```python
from build123d import *

# Parameters (mm, degrees)
F2_SIZE = 5
F3_R    = 0.99999


# Not quite as in the source:
# - a fillet or chamfer is up to 0.001 mm smaller than in the source, because OpenCascade refuses the exact size


with BuildPart() as f1:
    # F0 (on Front) → F1 (revolve)
    with BuildSketch(Plane.XZ):
        with BuildLine():
            Line((-2.5, -3), (-2.5, 0))
            Line((-2.5, 0), (-2.5, 15))
            Line((-2.5, 15), (-8, 15))
            ThreePointArc((-8, 15), (-11.5355339059, 13.5355339059), (-13, 10))
            Line((-13, 10), (-13, 8))
            Line((-13, 8), (-12, 8))
            ThreePointArc((-12, 8), (-8.4644660941, 6.5355339059), (-7, 3))
            ThreePointArc((-7, 3), (-7.8786796564, 0.8786796564), (-10, 0))
            Line((-10, 0), (-10.5, 0))
            Line((-10.5, 0), (-10.5, -3))
            Line((-10.5, -3), (-2.5, -3))
        make_face()
    revolve(axis=Axis((0, 0, 3.244361095), (0, 0, -1)))

    # F2
    f2_edges = [f1.edges().sort_by_distance(p)[0] for p in [
        (2.5, 0, 15),
    ]]
    chamfer(f2_edges, length=F2_SIZE)

    # F3 (radius 1 in the source; OpenCascade refuses exactly that, so slightly less here)
    f3_edges = [f1.edges().sort_by_distance(p)[0] for p in [
        (13, 0, 8),
    ]]
    fillet(f3_edges, radius=F3_R)


solid = f1.part
```
Here's how the part is built. I have some questions about the finished solid (model axes, mm). A direction names the side the tool comes from. Coordinates: 2 decimals unless noted, no trailing zeros. Write each loop counter-clockwise with the first axis right and the second up, starting at its lowest first coordinate (ties: lowest second). Pieces come first, ordered by that corner, then holes. Notation, with made-up numbers: M 17,78.25 L 35,78.25 A20 cw 35,86.25 Z; hole C 14,42.5 d4. An arc over 180 degrees is marked long. Answer as CSV lines item,"result". Start each with the question number.
Q1. Will these pins go through, and if not, where does the flat tip stop? pin 1 Ø2 at (y, z) = (-4, 0.5) entering from +X; pin 2 Ø8 at (x, z) = (6, 1.5) entering from -Y; pin 3 Ø3 at (x, y) = (-2.5, -5) entering from +Z.
Q2. If we mould it in two halves opening along Z, with no side actions, what happens to faces 1 (the flat face through (-2, -2, -3)), 2 (the flat face through (5, -9, 0)), 3 (the cylindrical face through (0.54, -2.44, 3.59))? For each: pulls with the +Z half, pulls with the -Z half, needs draft (parallel to the pull), parting line crosses it, or undercut.
Q3. Suppose I cut it at C-C, the plane z = -1. List the corners of the cut face in (x, y) for me, then the cut area to 3 significant figures.
Q4. Suppose I cut it at D-D, the plane z = 5.75. List the corners of the cut face in (x, y) for me, then the cut area to 3 significant figures.
Q5. For faces 4 (the cylindrical face through (-10, 3.2, -1.5)), 5 (the cylindrical face through (10.316, -7.91, 9.493)), which set-ups out of +Z, -Z, +X, -X, +Y, -Y let a thin tool reach every point of the face, with its end or its side?
Q6. I need wall thicknesses on probe 1 along Y at (x, z) = (0, 5.75); probe 2 along Z at (x, y) = (4.75, -9.25); probe 3 along Z at (x, y) = (9.25, 2.5). Which ranges of each line are inside material? Lowest first, please. Write a range as [from, to].
Entries:
1,pin 1,"stops at x = 10.02"
1,pin 2,"stops at y = -10.25"
1,pin 3,"stops at z = 14.59"
2,face 1,"pulls with the -Z half"
2,face 2,"undercut"
2,face 3,"needs draft"
3,outline,"C 0,0 d21; hole C 0,0 d5"
3,area,"327 mm²"
4,outline,"C 0,0 d15.65; hole C 0,0 d5"
4,area,"173 mm²"
5,face 4,"-Z"
5,face 5,"+Z, -Z"
6,probe 1,"y = [-7.82, -2.5], [2.5, 7.82]"
6,probe 2,"z = [-3, 0], [7.74, 14.39]"
6,probe 3,"z = [-3, 0.03], [7.38, 14.74]"
